The model under review builds one solid part; all positions refer to its coordinate system, in mm. Face numbers are marked on the shaded views. A direction names the side the tool comes from. Give positions to 0.01 mm unless a question says otherwise; leave off trailing zeros. Write each loop counter-clockwise with the first axis right and the second up, starting at its lowest first coordinate (ties: lowest second). Pieces come first, ordered by that corner, then holes.
from build123d import *

# Parameters (mm, degrees)
F0_R     = 12.5
F1_DEPTH = 25
F3_DEPTH = 12
F5_DEPTH = 25


with BuildPart() as f1:
    # F0 (on Top) → F1 (new body)
    with BuildSketch(Plane.XY):
        Circle(F0_R)
    extrude(amount=F1_DEPTH)

    # F2 (on face) → F3 (cut)
    with BuildSketch(Plane.XY.offset(25)):
        Polygon((-9.084021, -0.833007), (-3.820606, -8.283496), (5.263415, -7.450489), (9.084021, 0.833007), (3.820606, 8.283496), (-5.263415, 7.450489), align=None)
    extrude(amount=-F3_DEPTH, mode=Mode.SUBTRACT)

    # F4 (on face) → F5 (cut)
    with BuildSketch(Plane(origin=(0, 0, 0), x_dir=(1, 0, 0), z_dir=(0, 0, -1))):
        Polygon((0.158226, 4.522716), (-4.522716, 0.158226), (-0.158226, -4.522716), (4.522716, -0.158226), align=None)
    extrude(amount=-F5_DEPTH, mode=Mode.SUBTRACT)


solid = f1.part
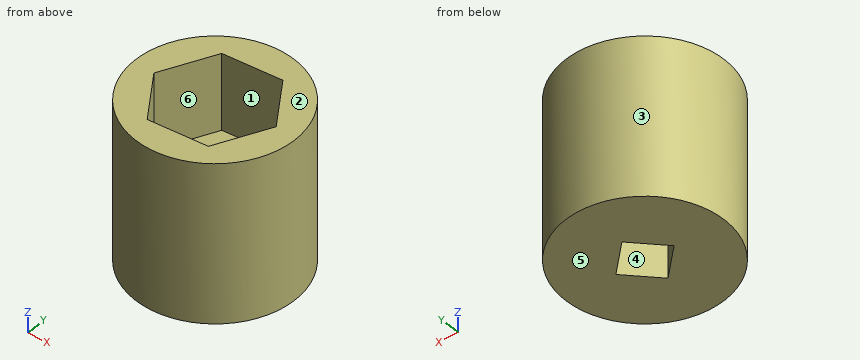
1) The part is to be moulded in two halves that separate along X. For the marked faces 1, 2 and 3, say which applies: +X half, -X half, draft (parallel to the pull), parting line (faces both ways), or undercut.
2) Insertion check: pin 1 (4 mm diameter, centred on x = -5.5, z = 19, fed in from +Y); pin 2 (2 mm diameter, centred on y = -6.5, z = 16.5, fed in from -X) (3 decimals); pin 3 (10 mm diameter, centred on y = -9.5, z = 4, fed in from -X). Each pin has a flat end and moves straight along its axis. Give the tip position at first contact, or say it passes through.
3) Consider section A-A, the plane z = 18.5. Give the boundary of the cut face in (x, y).
4) Tool access review of the marked faces 4, 5 and 6: name each direction out of +Z, -Z, +X, -X, +Y, -Y from which nothing blocks a thin tool from reaching the whole face with its end or side.
5) Consider section C-C, the plane y = 5.5. Give the boundary of the cut face in (x, z), then the cut area to 3 significant figures.
6) To check wall thickness, follow probe 1 along Y at (x, z) = (-1, 2.25); probe 2 along Y at (x, z) = (-2, 7); probe 3 along X at (y, z) = (2.75, 4). State the ranges of each line that lie inside material, in increasing order.
7) Consider section B-B, the plane x = 1. Give the boundary of the cut face in (y, z), then the cut area to 3 significant figures.
8) Consider section D-D, the plane x = 10. Give the boundary of the cut face in (y, z), then the cut area to 3 significant figures.
Answer block:
1. face 1: undercut
1. face 2: draft
1. face 3: parting line
2. pin 1: stops at y = 12
2. pin 2: stops at x = -11.225
2. pin 3: stops at x = -11.66
3. outline: circle Ø25 at (0, 0); hole (-9.08, -0.83) - (-3.82, -8.28) - (5.26, -7.45) - (9.08, 0.83) - (3.82, 8.28) - (-5.26, 7.45) - close
4. face 4: +Z, -Z
4. face 5: -Z, +X, -X, +Y, -Y
4. face 6: +Z
5. outline: (-11.22, 0) - (11.22, 0) - (11.22, 25) - (5.79, 25) - (5.79, 13) - (-6.16, 13) - (-6.16, 25) - (-11.22, 25) - close
5. area: 418 mm2
6. probe 1: y = -12.46 to -3.44, 3.62 to 12.46
6. probe 2: y = -12.34 to -2.51, 2.55 to 12.34
6. probe 3: x = -12.19 to -1.81, 1.74 to 12.19
7. outline: (-12.46, 0) - (-3.62, 0) - (-3.62, 13) - (-7.84, 13) - (-7.84, 25) - (-12.46, 25) - close; (3.44, 0) - (12.46, 0) - (12.46, 25) - (8.02, 25) - (8.02, 13) - (3.44, 13) - close
7. area: 341 mm2
8. outline: (-7.5, 0) - (7.5, 0) - (7.5, 25) - (-7.5, 25) - close
8. area: 375 mm2
